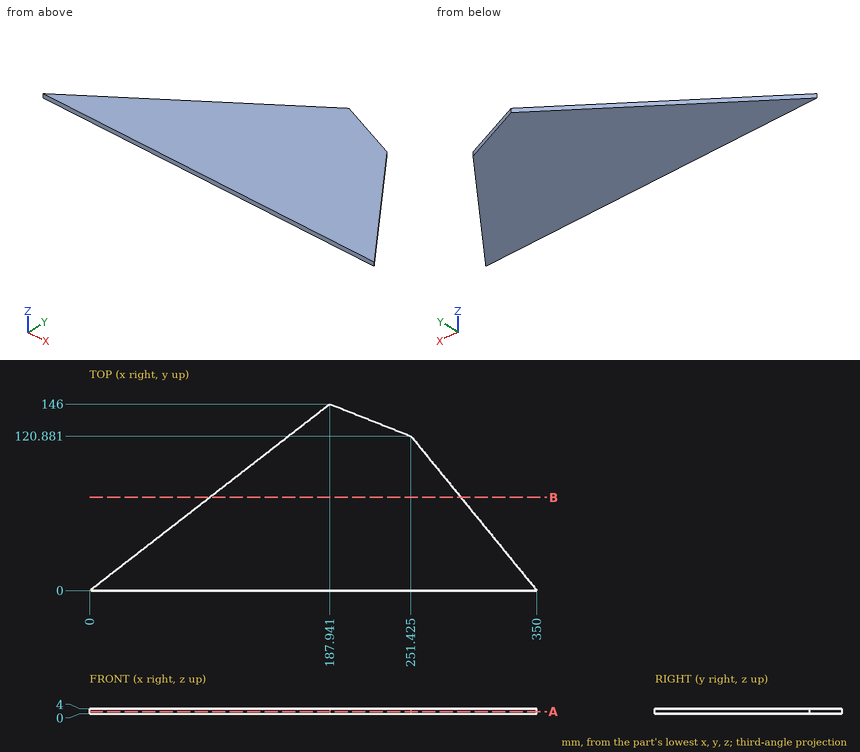
Could you check a few things on this drawing? It's one solid part, dimensions in mm from its lowest x, y, z. Coordinates: 2 decimals unless noted, no trailing zeros. Order: outer loops, then holes, each group sorted by start corner. A loop starts at its lowest first (then second) coordinate and runs counter-clockwise, first axis right, second up.
1) Imagine slicing it at A-A on z = 1.65. List the corners of the cut face in (x, y) for me (1 decimal).
2) Imagine slicing it at B-B on y = 73. List the corners of the cut face in (x, z) for me, and give its area (3 significant figures).
3) I need wall thicknesses on line 1 (Y direction, x = 154, z = 0.85); line 2 (Y direction, x = 304, z = 2.95); line 3 (X direction, y = 27, z = 0.2) (1 decimal). Which ranges of each line are inside material? Lowest first, please.
Response values:
1. outline: (0, 0) - (350, 0) - (251.4, 120.9) - (187.9, 146) - close
2. outline: (93.97, 0) - (290.47, 0) - (290.47, 4) - (93.97, 4) - close
2. area: 786 mm2
3. line 1: y = 0 to 119.63
3. line 2: y = 0 to 56.41
3. line 3: x = 34.8 to 328
